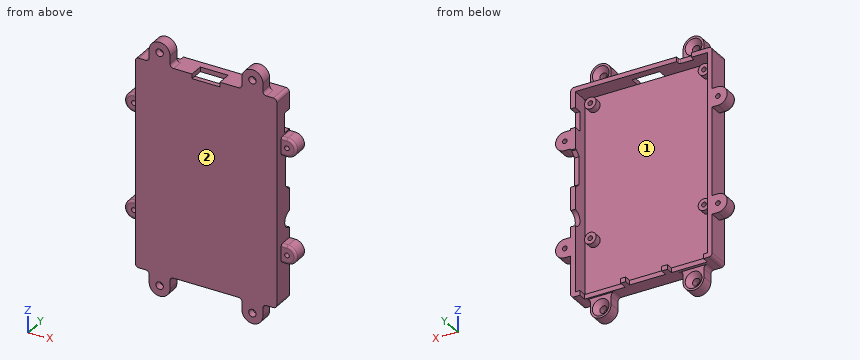
from build123d import *

# Parameters (mm, degrees)
SKETCH_1_W               = 61
SKETCH_1_H               = 90
EXTRUDE_461_DEPTH        = 9.2
SKETCH_2_W               = 57
SKETCH_2_H               = 86
CUT_EXTRUDE_685_DEPTH    = 7.2
SKETCH_3_R               = 2.5
SKETCH_3_R_2             = 1
EXTRUDE_939_DEPTH        = 3
SKETCH_4_W               = 8.5
SKETCH_4_H               = 4
MICROUSB_DEPTH           = 2
SKETCH_5_W               = 16
SKETCH_5_H               = 6.05
HDMI_DEPTH               = 2
SKETCH_6_R               = 3.5
CUT_EXTRUDE_1702_DEPTH   = 2
SKETCH_7_W               = 17.5
SKETCH_7_H               = 14
ETHERNET_DEPTH           = 2
SKETCH_8_W               = 15.5
SKETCH_8_H               = 16.12
USB_DEPTH                = 2
PATTERN_LINEAR_1_COUNT   = 2
PATTERN_LINEAR_1_PITCH   = 18
SKETCH_9_W               = 12
SKETCH_9_H               = 6
MICROSD_DEPTH            = 2
SKETCH_10_R              = 1.6
EXTRUDE_2923_DEPTH       = 5
MIRROR_2_COPY_1_SKETCH_R = 1.6
MIRROR_2_COPY_1_DEPTH    = 5
SKETCH_11_R              = 1
EXTRUDE_3371_DEPTH       = 6
MIRROR_4_COPY_1_SKETCH_R = 1
MIRROR_4_COPY_1_DEPTH    = 6
CHAMFER_1_SIZE           = 2
FILLET_1_R               = 1
FILLET_2_R               = 1.5
SKETCH_12_W              = 6.3
SKETCH_12_H              = 2
CUT_EXTRUDE_5754_DEPTH   = 2
FILLET_3_R               = 0.5
CHAMFER_2_SIZE           = 2


with BuildPart() as part:
    # Эскиз1 → Extrude 461 (new body)
    with BuildSketch(Plane(origin=(0, 0, 0), x_dir=(1, 0, 0), z_dir=(0, 1, 0))):
        Rectangle(SKETCH_1_W, SKETCH_1_H)
    extrude(amount=EXTRUDE_461_DEPTH)

    # Эскиз2 → Cut-Extrude 685 (cut)
    with BuildSketch(Plane(origin=(0, 9.2, 0), x_dir=(1, 0, 0), z_dir=(0, 1, 0))):
        Rectangle(SKETCH_2_W, SKETCH_2_H)
    extrude(amount=-CUT_EXTRUDE_685_DEPTH, mode=Mode.SUBTRACT)

    # Эскиз3 → Extrude 939 (add)
    # profile 1 of 4: a face of its own
    with BuildSketch(Plane(origin=(0, 2, 0), x_dir=(1, 0, 0), z_dir=(0, 1, 0))):
        with Locations(Location((-24.5, 19, 0), (0, 0, 270))):
            Circle(SKETCH_3_R)
        with Locations(Location((-24.5, 19, 0), (0, 0, 270))):
            Circle(SKETCH_3_R_2, mode=Mode.SUBTRACT)
    # profile 2 of 4: a face of its own
    with BuildSketch(Plane(origin=(0, 2, 0), x_dir=(1, 0, 0), z_dir=(0, 1, 0))):
        with Locations(Location((24.5, 19, 0), (0, 0, 270))):
            Circle(SKETCH_3_R)
        with Locations(Location((24.5, 19, 0), (0, 0, 270))):
            Circle(SKETCH_3_R_2, mode=Mode.SUBTRACT)
    # profile 3 of 4: a face of its own
    with BuildSketch(Plane(origin=(0, 2, 0), x_dir=(1, 0, 0), z_dir=(0, 1, 0))):
        with Locations(Location((24.5, -39, 0), (0, 0, 270))):
            Circle(SKETCH_3_R)
        with Locations(Location((24.5, -39, 0), (0, 0, 270))):
            Circle(SKETCH_3_R_2, mode=Mode.SUBTRACT)
    # profile 4 of 4: a face of its own
    with BuildSketch(Plane(origin=(0, 2, 0), x_dir=(1, 0, 0), z_dir=(0, 1, 0))):
        with Locations(Location((-24.5, -39, 0), (0, 0, 270))):
            Circle(SKETCH_3_R)
        with Locations(Location((-24.5, -39, 0), (0, 0, 270))):
            Circle(SKETCH_3_R_2, mode=Mode.SUBTRACT)
    extrude(amount=EXTRUDE_939_DEPTH)

    # Эскиз4 → microusb (cut)
    with BuildSketch(Plane(origin=(30.5, 0, 0), x_dir=(0, 0, -1), z_dir=(1, 0, 0))):
        with Locations((-31.9, 7.7)):
            Rectangle(SKETCH_4_W, SKETCH_4_H)
    extrude(amount=-MICROUSB_DEPTH, mode=Mode.SUBTRACT)

    # Эскиз5 → hdmi (cut)
    with BuildSketch(Plane(origin=(30.5, 0, 0), x_dir=(0, 0, -1), z_dir=(1, 0, 0))):
        with Locations((-10.5, 9.405)):
            Rectangle(SKETCH_5_W, SKETCH_5_H)
    extrude(amount=-HDMI_DEPTH, mode=Mode.SUBTRACT)

    # Эскиз6 → Cut-Extrude 1702 (cut)
    with BuildSketch(Plane(origin=(30.5, 0, 0), x_dir=(0, 0, -1), z_dir=(1, 0, 0))):
        with Locations((11, 9.3)):
            Circle(SKETCH_6_R)
    extrude(amount=-CUT_EXTRUDE_1702_DEPTH, mode=Mode.SUBTRACT)

    # Эскиз7 → ethernet (cut)
    with BuildSketch(Plane(origin=(0, 0, -45), x_dir=(-1, 0, 0), z_dir=(0, 0, -1))):
        with Locations((-17.75, 12.75)):
            Rectangle(SKETCH_7_W, SKETCH_7_H)
    extrude(amount=-ETHERNET_DEPTH, mode=Mode.SUBTRACT)

    # Эскиз8 → usb (cut)
    with BuildSketch(Plane(origin=(0, 0, -45), x_dir=(-1, 0, 0), z_dir=(0, 0, -1))):
        with Locations((1, 14.39)):
            Rectangle(SKETCH_8_W, SKETCH_8_H)
    usb = extrude(amount=-USB_DEPTH, mode=Mode.SUBTRACT)

    # Линейный массив1: usb ×2
    with Locations(*[(-i * PATTERN_LINEAR_1_PITCH, 0, 0) for i in range(1, PATTERN_LINEAR_1_COUNT)]):
        add(usb, mode=Mode.SUBTRACT)

    # Эскиз9 → microsd (cut)
    with BuildSketch(Plane.XY.offset(45)):
        with Locations((0, 3)):
            Rectangle(SKETCH_9_W, SKETCH_9_H)
    extrude(amount=-MICROSD_DEPTH, mode=Mode.SUBTRACT)

    # Эскиз10 → Extrude 2923 (add)
    with BuildSketch(Plane.XZ):
        with BuildLine():
            Line((-24.5, 50), (-24.5, 45))
            Line((-24.5, 45), (-15.5, 45))
            Line((-15.5, 45), (-15.5, 50))
            ThreePointArc((-15.5, 50), (-20, 54.5), (-24.5, 50))
        make_face()
        with Locations(Location((-20, 50, 0), (0, 0, 270))):
            Circle(SKETCH_10_R, mode=Mode.SUBTRACT)
    extrude_2923 = extrude(amount=-EXTRUDE_2923_DEPTH)

    # Зеркальное отражение1: Extrude 2923 across plane
    add(extrude_2923.mirror(Plane(origin=(0, 0, 0), x_dir=(0, 0, 1), z_dir=(1, 0, 0))))

    # Зеркальное отражение2: Extrude 2923 across plane
    add(extrude_2923.mirror(Plane.XY))

    # Зеркальное отражение2 copy 1 sketch → Зеркальное отражение2 copy 1 (add)
    with BuildSketch(Plane(origin=(0, 0, 0), x_dir=(-1, 0, 0), z_dir=(0, -1, 0))):
        with BuildLine():
            Line((-24.5, 50), (-24.5, 45))
            Line((-24.5, 45), (-15.5, 45))
            Line((-15.5, 45), (-15.5, 50))
            ThreePointArc((-15.5, 50), (-20, 54.5), (-24.5, 50))
        make_face()
        with Locations(Location((-20, 50, 0), (0, 0, 270))):
            Circle(MIRROR_2_COPY_1_SKETCH_R, mode=Mode.SUBTRACT)
    extrude(amount=-MIRROR_2_COPY_1_DEPTH)

    # Эскиз11 → Extrude 3371 (add)
    with BuildSketch(Plane(origin=(0, 9.2, 0), x_dir=(1, 0, 0), z_dir=(0, 1, 0))):
        with BuildLine():
            Line((-33, 27), (-30.5, 27))
            Line((-30.5, 27), (-30.5, 19))
            Line((-30.5, 19), (-33, 19))
            ThreePointArc((-33, 19), (-37, 23), (-33, 27))
        make_face()
        with Locations(Location((-33, 23, 0), (0, 0, 270))):
            Circle(SKETCH_11_R, mode=Mode.SUBTRACT)
    extrude_3371 = extrude(amount=-EXTRUDE_3371_DEPTH)

    # Зеркальное отражение3: Extrude 3371 across plane
    add(extrude_3371.mirror(Plane(origin=(0, 0, 0), x_dir=(0, 0, 1), z_dir=(1, 0, 0))))

    # Зеркальное отражение4: Extrude 3371 across plane
    add(extrude_3371.mirror(Plane.XY))

    # Зеркальное отражение4 copy 1 sketch → Зеркальное отражение4 copy 1 (add)
    with BuildSketch(Plane(origin=(0, 9.2, 0), x_dir=(-1, 0, 0), z_dir=(0, 1, 0))):
        with BuildLine():
            Line((-33, 27), (-30.5, 27))
            Line((-30.5, 27), (-30.5, 19))
            Line((-30.5, 19), (-33, 19))
            ThreePointArc((-33, 19), (-37, 23), (-33, 27))
        make_face()
        with Locations(Location((-33, 23, 0), (0, 0, 270))):
            Circle(MIRROR_4_COPY_1_SKETCH_R, mode=Mode.SUBTRACT)
    extrude(amount=-MIRROR_4_COPY_1_DEPTH)

    # Фаска1
    chamfer_1_edges = [part.edges().sort_by_distance(p)[0] for p in [
        (29.5, 6.38, 18.5),
        (29.5, 6.38, 2.5),
    ]]
    chamfer(chamfer_1_edges, length=CHAMFER_1_SIZE)

    # Скругление1
    fillet_1_edges = [part.edges().sort_by_distance(p)[0] for p in [
        (-37, 3.2, -23),
        (-31.75, 3.2, -27),
        (-31.75, 3.2, -19),
        (37, 3.2, -23),
        (31.75, 3.2, -19),
        (31.75, 3.2, -27),
        (37, 3.2, 23),
        (31.75, 3.2, 27),
        (31.75, 3.2, 19),
        (-37, 3.2, 23),
        (-31.75, 3.2, 19),
        (-31.75, 3.2, 27),
    ]]
    fillet(fillet_1_edges, radius=FILLET_1_R)

    # Скругление2
    fillet_2_edges = [part.edges().sort_by_distance(p)[0] for p in [
        (-15.5, 2.5, 45),
        (-24.5, 2.5, 45),
        (24.5, 2.5, 45),
        (15.5, 2.5, 45),
        (15.5, 2.5, -45),
        (24.5, 2.5, -45),
        (-24.5, 2.5, -45),
        (-15.5, 2.5, -45),
        (-30.5, 4.6, -45),
        (30.5, 4.6, -45),
        (30.5, 4.6, 45),
        (-30.5, 4.6, 45),
    ]]
    fillet(fillet_2_edges, radius=FILLET_2_R)

    # Эскиз12 → Cut-Extrude 5754 (cut)
    with BuildSketch(Plane.XY.offset(45)):
        with Locations((-18.35, 8.2)):
            Rectangle(SKETCH_12_W, SKETCH_12_H)
    extrude(amount=-CUT_EXTRUDE_5754_DEPTH, mode=Mode.SUBTRACT)

    # Скругление3
    fillet_3_edges = [part.edges().sort_by_distance(p)[0] for p in [
        (-21.5, 7.2, 44),
        (-15.2, 7.2, 44),
    ]]
    fillet(fillet_3_edges, radius=FILLET_3_R)

    # Фаска2
    chamfer_2_edges = [part.edges().sort_by_distance(p)[0] for p in [
        (-20, 5, 51.6),
        (20, 5, 51.6),
        (20, 5, -51.6),
        (-20, 5, -51.6),
    ]]
    chamfer(chamfer_2_edges, length=CHAMFER_2_SIZE)


solid = part.part
Design review of the part built by this model. Coordinates are the model's own, in mm. Face numbers are marked on the shaded views. Round coordinates to 2 decimals unless told otherwise and drop trailing zeros. Order: outer loops, then holes, each group sorted by start corner. A loop starts at its lowest first (then second) coordinate and runs counter-clockwise, first axis right, second up.
1) Consider section B-B (z = 31). State the section outline as (x, y) points.
The answers:
outline: (-30.5, 0) - (30.5, 0) - (30.5, 5.7) - (28.5, 5.7) - (28.5, 2) - (-28.5, 2) - (-28.5, 9.2) - (-30.5, 9.2) - close
2) Consider section C-C (z = -12). State the section outline as (x, y) points.
The answers:
outline: (-30.5, 0) - (30.5, 0) - (30.5, 5.95) - (28.5, 5.95) - (28.5, 2) - (-28.5, 2) - (-28.5, 9.2) - (-30.5, 9.2) - close
3) Draft analysis for pull direction X (two halves, no side actions). For the marked faces 1 and 2, state which applies: released by +X, released by -X, zero draft, split by the parting line, or undercut.
The answers:
face 1: undercut
face 2: zero draft
4) Consider section A-A (x = -4.5). State the section outline as (y, z) points, plus the area to 3 significant figures.
The answers:
outline: (0, -45) - (6.33, -45) - (6.33, -43) - (2, -43) - (2, 43) - (0, 43) - close; (6, 43) - (9.2, 43) - (9.2, 45) - (6, 45) - close
area: 191 mm2
5) Clearance check with flat-ended pins moving along their axes: pin 1 Ø5 at (x, y) = (24.5, 1.5) entering from -Z; pin 2 Ø17 at (x, z) = (13.5, -2) entering from +Y; pin 3 Ø5 at (y, z) = (4.5, 40) entering from +X; pin 4 Ø3 at (x, z) = (-20, 50) entering from +Y. State where each tip first meets the part, or that it passes through.
The answers:
pin 1: stops at z = -54.03
pin 2: stops at y = 2
pin 3: stops at x = 30.5
pin 4: passes through
6) For L1, parallel to Z at x = 20, y = 1.2; L2, parallel to X at y = 3.2, z = -19; L3, parallel to Z at x = 33, y = 6.5, list the stretches that pass through material, from the lowest coordinate up.
The answers:
L1: z = -54.5 to -51.6, -48.4 to 48.4, 51.6 to 54.5
L2: x = -30.5 to -28.5, -27 to -25.5, -23.5 to -22, 22 to 23.5, 25.5 to 27, 28.5 to 30.5
L3: z = -27 to -24, -22 to -19, 19 to 22, 24 to 27
